```python
from build123d import *

# Parameters (mm, degrees)
CROQUIS1_W              = 95
CROQUIS1_H              = 50
SALIENTE_EXTRUIR1_DEPTH = 10
CROQUIS2_W              = 21
CROQUIS2_H              = 4.123726598
CORTAR_EXTRUIR1_DEPTH   = 20
CORTAR_EXTRUIR2_DEPTH   = 1000
REDONDEO1_R             = 5
CROQUIS5_R              = 1.5
CORTAR_EXTRUIR3_DEPTH   = 10
CORTAR_EXTRUIR4_DEPTH   = 140
CROQUIS8_W              = 21.19141069
CROQUIS8_H              = 3.071218941
CROQUIS8_W_2            = 21.2
CORTAR_EXTRUIR5_DEPTH   = 5
REDONDEO2_R             = 10
REDONDEO3_R             = 10
CROQUIS9_W              = 95
CROQUIS9_H              = 3.240818253
SALIENTE_EXTRUIR2_DEPTH = 10
REDONDEO4_R             = 5


with BuildPart() as part:
    # Croquis1 → Saliente-Extruir1 (new body)
    with BuildSketch(Plane.XY):
        with Locations((0.195712782, 7.120478413)):
            Rectangle(CROQUIS1_W, CROQUIS1_H)
    extrude(amount=SALIENTE_EXTRUIR1_DEPTH)

    # Croquis2 → Cortar-Extruir1 (cut)
    with BuildSketch(Plane.XY.offset(10)):
        with Locations((-21.804287218, -10.817658288)):
            Rectangle(CROQUIS2_W, CROQUIS2_H)
        with Locations((22.195712782, -10.817658288)):
            Rectangle(CROQUIS2_W, CROQUIS2_H)
    extrude(amount=-CORTAR_EXTRUIR1_DEPTH, mode=Mode.SUBTRACT)

    # Croquis3 → Cortar-Extruir2 (cut)
    with BuildSketch(Plane.ZY.offset(47.304287218)):
        Polygon((0, -17.879521587), (10, -4.774745355), (10, -17.879521587), align=None)
    extrude(amount=-CORTAR_EXTRUIR2_DEPTH, mode=Mode.SUBTRACT)

    # Redondeo1
    redondeo1_edges = [part.edges().sort_by_distance(p)[0] for p in [
        (0.195712782, 32.120478413, 10),
    ]]
    fillet(redondeo1_edges, radius=REDONDEO1_R)

    # Croquis5 → Cortar-Extruir3 (cut)
    with BuildSketch(Plane.XY.offset(10)):
        with Locations((-39.804287218, 15.480478413)):
            Circle(CROQUIS5_R)
        with Locations(Location((40.195712782, 15.480478413, 0), (0, 0, 180))):
            Circle(CROQUIS5_R)
        with Locations((-13.357848867, -2.379521587)):
            Circle(CROQUIS5_R)
        with Locations(Location((13.749274431, -2.379521587, 0), (0, 0, 180))):
            Circle(CROQUIS5_R)
        with Locations((-39.804287218, -2.859521587)):
            Circle(CROQUIS5_R)
        with Locations(Location((40.195712782, -2.859521587, 0), (0, 0, 180))):
            Circle(CROQUIS5_R)
    extrude(amount=-CORTAR_EXTRUIR3_DEPTH, mode=Mode.SUBTRACT)

    # Croquis7 → Cortar-Extruir4 (cut)
    with BuildSketch(Plane.ZY.offset(47.304287218)):
        Polygon((10, -4.774745355), (4.790814809, -4.774745355), (3.240818253, -4.774745355), (3.240818253, -4.292734616), (3.240818253, 32.120478413), (5, 32.120478413), (10, 32.120478413), align=None)
    extrude(amount=-CORTAR_EXTRUIR4_DEPTH, mode=Mode.SUBTRACT)

    # Croquis8 → Cortar-Extruir5 (cut)
    with BuildSketch(Plane(origin=(0, -4.774745355, 0), x_dir=(1, 0, 0), z_dir=(0, 1, 0))):
        with Locations((-21.763502643, -6.820936578)):
            Rectangle(CROQUIS8_W, CROQUIS8_H)
        with Locations((22.159222862, -6.820936578)):
            Rectangle(CROQUIS8_W_2, CROQUIS8_H)
    extrude(amount=-CORTAR_EXTRUIR5_DEPTH, mode=Mode.SUBTRACT)

    # Redondeo2
    # the kernel refuses this fillet: 10 mm, written as the material it takes off along each edge
    with BuildSketch(Plane(origin=(-11.304287218, -8.755794989, 5.285327107), x_dir=(0, 0, -1), z_dir=(-1, 0, 0))) as redondeo2_piece_1:
        with BuildLine():
            CenterArc((10, -8.818835496), REDONDEO2_R, 118.129583681, 61.870416319)
            Line((0, -8.818835496), (-0.2, -8.818835496))
            Line((-0.2, -8.818835496), (-0.2, 0))
            Line((-0.2, 0), (0, 0.2))
            ThreePointArc((0, 0.2), (2.642663554, 0.2), (5.191033649, 0.17637671))
            Line((5.191033649, 0.17637671), (5.285327107, 0))
        make_face()
    extrude(amount=21, mode=Mode.SUBTRACT)

    # Redondeo3
    # the kernel refuses this fillet: 10 mm, written as the material it takes off along each edge
    with BuildSketch(Plane(origin=(11.695712782, -8.755794989, 5.285327107), x_dir=(0, 0, -1), z_dir=(1, 0, 0))) as redondeo3_piece_1:
        with BuildLine():
            CenterArc((10, 8.818835496), REDONDEO3_R, 180, 61.870416319)
            Line((0, 8.818835496), (-0.2, 8.818835496))
            Line((-0.2, 8.818835496), (-0.2, 0))
            Line((-0.2, 0), (0, -0.2))
            ThreePointArc((0, -0.2), (2.642663554, -0.2), (5.191033649, -0.17637671))
            Line((5.191033649, -0.17637671), (5.285327107, 0))
        make_face()
    extrude(amount=21, mode=Mode.SUBTRACT)

    # Croquis9 → Saliente-Extruir2 (add)
    with BuildSketch(Plane(origin=(0, 32.120478413, 0), x_dir=(1, 0, 0), z_dir=(0, 1, 0))):
        with Locations((0.195712782, -1.620409127)):
            Rectangle(CROQUIS9_W, CROQUIS9_H)
    extrude(amount=SALIENTE_EXTRUIR2_DEPTH)

    # Redondeo4
    # the kernel refuses this fillet: 5 mm, written as the material it takes off along each edge
    with BuildSketch(Plane(origin=(59.396481876, 42.120478413, 3.240818253), x_dir=(0, 0, -1), z_dir=(-1, 0, 0))) as redondeo4_piece_1:
        with BuildLine():
            CenterArc((5, 4.680307637), REDONDEO4_R, 180, 69.400324349)
            Line((0, 4.680307637), (-0.1, 4.680307637))
            Line((-0.1, 4.680307637), (-0.1, 0))
            Line((-0.1, 0), (0, -0.1))
            ThreePointArc((0, -0.1), (1.620409126, -0.1), (3.205634618, -0.093606153))
            Line((3.205634618, -0.093606153), (3.240818253, 0))
        make_face()
    extrude(amount=118.401538187, mode=Mode.SUBTRACT)


solid = part.part
```
Check sheet for the modelled part. Datum: model origin and axes. Units: mm. A direction names the side the tool comes from. Round coordinates to 2 decimals unless told otherwise and drop trailing zeros. Order: outer loops, then holes, each group sorted by start corner. A loop starts at its lowest first (then second) coordinate and runs counter-clockwise, first axis right, second up. Notation, with made-up numbers: (-5, 54.5) -> (52, 54.5) arc R14 ccw to (52, 60.5) -> close; hole circle Ø7 at (38, 36.5). An arc over 180 degrees is marked (long way). One line per item, written item: value. Start each with the question number.
Q1. Cross-section at B-B (z = 7.25). Record the boundary of the cut face in (x, y), and give its area (3 significant figures).
Q2. Thickness scan on line 1 (Z direction, x = 44, y = 28); line 2 (Y direction, x = 28, z = 2.25); line 3 (Y direction, x = -21.5, z = 2.5). Record the ranges inside material, lowest first.
Q3. Set-up check for faces 4 (the face through (0, 16, 3.241)), 5 (the face through (22, -12.88, 2)), 6 (the face through (-21.657, -7.086, 2.278)): record each of +Z, -Z, +X, -X, +Y, -Y from which the full face is reachable in a straight line by a thin tool's end or side.
Q4. Gauge pin test, flat ends, axial feed: pin 1 Ø2 at (x, z) = (-7, 6) entering from +Y; pin 2 Ø4 at (x, z) = (0, 1) entering from +Y; pin 3 Ø8 at (x, y) = (13.5, 1) entering from +Z; pin 4 Ø4 at (y, z) = (-10, 6.5) entering from +X. Record the tip position at first contact, or that the pin passes through.
Q5. Cross-section at C-C (x = -1.5). Record the boundary of the cut face in (y, z), and give its area (3 significant figures).
Q6. Cross-section at D-D (z = 1.25). Give the number of separate pieces and of enclosed holes in the cut face, and give its area (3 significant figures).
Q7. Mould release check, pull along Y, two halves, no side actions. Record for faces 1 (the face through (0, -4.775, 7)), 2 (the face through (0, 12, 0)), 3 (the face through (-11.304, -10, 3)): pulls with the +Y half, pulls with the -Y half, needs draft (parallel to the pull), parting line crosses it, or undercut.
Q8. Cross-section at A-A (x = 27.5). Record the boundary of the cut face in (y, z), and give its area (3 significant figures).
Completed:
1. outline: (-47.3, -8.38) -> (-32.36, -8.38) -> (-32.36, -4.77) -> (-47.3, -4.77) -> close; (-11.17, -8.38) -> (11.56, -8.38) -> (11.56, -4.77) -> (-11.17, -4.77) -> close; (32.76, -8.38) -> (47.7, -8.38) -> (47.7, -4.77) -> (32.76, -4.77) -> close
1. area: 190 mm²
2. line 1: z = 0 to 3.24
2. line 2: y = -14.93 to -12.88, -7.11 to 40.43
2. line 3: y = -14.6 to -12.88, -6.86 to 40.06
3. face 4: +Z, +X, -X, +Y
3. face 5: +Z, -Z
3. face 6: none
4. pin 1: stops at y = -4.77
4. pin 2: stops at y = 42.12
4. pin 3: stops at z = 3.24
4. pin 4: stops at x = 47.7
5. outline: (-17.88, 0) -> (42.12, 0) arc R5 ccw to (37.44, 3.24) -> (-4.77, 3.24) -> (-4.77, 10) -> close
5. area: 213 mm²
6. separate pieces: 1
6. enclosed holes: 8
6. area: 5,230 mm²
7. face 1: pulls with the +Y half
7. face 2: needs draft
7. face 3: undercut
8. outline: (-17.88, 0) -> (-12.88, 0) -> (-12.88, 3.82) -> close; (-8.76, 0) -> (42.12, 0) arc R5 ccw to (37.44, 3.24) -> (-4.77, 3.24) -> (-4.77, 4.04) arc R10 ccw to start; (-6.93, 8.36) -> (-4.77, 8.36) -> (-4.77, 10) -> close
8. area: 169 mm²
